from build123d import *

# Parameters (mm, degrees)
SKETCH1_W                      = 40
SKETCH1_H                      = 100
SKETCH1_W_2                    = 34
SKETCH1_H_2                    = 94
BOSS_EXTRUDE1_DEPTH            = 232.9
CUT_EXTRUDE2_REACH             = 283.987
SKETCH8_W                      = 34
SKETCH8_H                      = 16
CUT_EXTRUDE2_DIRECTION_2_DEPTH = 282.986542232
M4_CLEARANCE_HOLE1_D           = 4.5
M4_CLEARANCE_HOLE1_ON_FACE_2_D = 4.5
M4_CLEARANCE_HOLE1_ON_FACE_3_D = 4.5
M4_CLEARANCE_HOLE1_ON_FACE_4_D = 4.5
FILLET1_R                      = 2
F_3_0_3_DIAMETER_HOLE1_D       = 3
F_3_0_3_DIAMETER_HOLE1_DEPTH   = 3


with BuildPart() as part:
    # Sketch1 → Boss-Extrude1 (new body)
    with BuildSketch(Plane.XY.offset(30)):
        Rectangle(SKETCH1_W, SKETCH1_H)
        Rectangle(SKETCH1_W_2, SKETCH1_H_2, mode=Mode.SUBTRACT)
    extrude(amount=BOSS_EXTRUDE1_DEPTH)

    # Sketch8 → Cut-Extrude2 (cut, up to next)
    with BuildSketch(Plane(origin=(0, 50, 0), x_dir=(1, 0, 0), z_dir=(0, 1, 0)), mode=Mode.PRIVATE) as cut_extrude2_sk1:
        with Locations((0, -254.9)):
            Rectangle(SKETCH8_W, SKETCH8_H)
    cut_extrude2_tool1 = extrude(cut_extrude2_sk1.sketch, amount=-CUT_EXTRUDE2_REACH, mode=Mode.PRIVATE) & part.part
    add(cut_extrude2_tool1.solids().sort_by_distance((0, 50, 254.9))[0], mode=Mode.SUBTRACT)

    # Sketch8 → Cut-Extrude2 direction 2 (cut)
    with BuildSketch(Plane(origin=(0, 50, 0), x_dir=(1, 0, 0), z_dir=(0, 1, 0))):
        with Locations((0, -254.9)):
            Rectangle(SKETCH8_W, SKETCH8_H)
    extrude(amount=CUT_EXTRUDE2_DIRECTION_2_DEPTH, mode=Mode.SUBTRACT)

    # M4 Clearance Hole1 (through all)
    with Locations(Plane(origin=(20, 37, 37.5), x_dir=(0, 0, 1), z_dir=(1, 0, 0))):
        with Locations((0, 0), (0, 37), (217.9, 68), (217.9, 31.7), (217.9, -4.6), (0, 74)):
            Hole(M4_CLEARANCE_HOLE1_D / 2)

    # M4 Clearance Hole1 on face 2 (through all)
    with Locations(Plane(origin=(0, 50, 37.5), x_dir=(0, 0, 1), z_dir=(0, 1, 0))):
        with Locations((0, 0)):
            Hole(M4_CLEARANCE_HOLE1_ON_FACE_2_D / 2)

    # M4 Clearance Hole1 on face 3 (through all)
    with Locations(Plane(origin=(-20, -37, 37.5), x_dir=(0, 0, -1), z_dir=(-1, 0, 0))):
        with Locations((0, 0), (0, -37), (0, -74), (-217.9, -6), (-217.9, -42.3), (-217.9, -78.6)):
            Hole(M4_CLEARANCE_HOLE1_ON_FACE_3_D / 2)

    # M4 Clearance Hole1 on face 4 (through all)
    with Locations(Plane(origin=(0, -50, 37.5), x_dir=(0, 0, -1), z_dir=(0, -1, 0))):
        with Locations((0, 0), (-217.9, 0)):
            Hole(M4_CLEARANCE_HOLE1_ON_FACE_4_D / 2)

    # Fillet1
    fillet1_edges = [part.edges().sort_by_distance(p)[0] for p in [
        (17, 48.5, 246.9),
        (-17, 48.5, 246.9),
    ]]
    fillet(fillet1_edges, radius=FILLET1_R)

    # Ø3.0 (3) Diameter Hole1
    with Locations(Plane(origin=(20, 0, 0), x_dir=(0, 0, -1), z_dir=(1, 0, 0))):
        with Locations((-56.45, -45), (-236.45, -39), (-236.45, -45), (-191.45, -39), (-146.45, -39), (-101.45, -39), (-56.45, -39), (-191.45, -45), (-146.45, -45), (-101.45, -45)):
            Hole(F_3_0_3_DIAMETER_HOLE1_D / 2, depth=F_3_0_3_DIAMETER_HOLE1_DEPTH)


solid = part.part
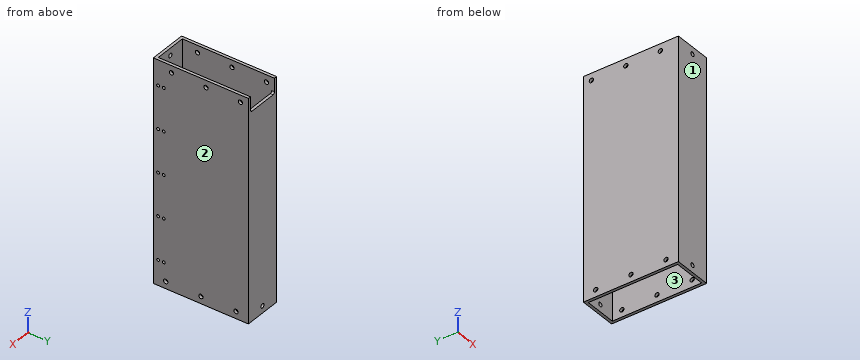
For this review, take the finished solid that the model builds, in its own axes (mm). Face numbers are marked on the shaded views. Give positions to 0.01 mm unless a question says otherwise; leave off trailing zeros. Loops run counter-clockwise (first coordinate to the right, second up) from the corner with the lowest first, then second, coordinate; pieces in that order, holes last. Notation, with made-up numbers: M -14,45.5 L 37,45.5 A17 cw 37,66.5 Z; hole C -16,47 d3. An arc over 180 degrees is marked long. Put each result on its own line as item: value. Start each with the question number.
(1) Wall thickness on L1, parallel to Y at x = 19, z = 255; L2, parallel to X at y = 11, z = 106; L3, parallel to Y at x = -16, z = 216: over which ranges is each line inside the solid? List them lowest first.
(2) Add section C-C, the plane z = 124. Write out the cut boundary in (x, y).
(3) Add section D-D, the plane y = -20. Write out the cut boundary in (x, z).
(4) The part is to be moulded in two halves that separate along Y. For the marked faces 1, 2 and 3, say which applies: +Y half, -Y half, draft (parallel to the pull), parting line (faces both ways), or undercut.
(5) Add section A-A, the plane x = 11.5. Write out the cut boundary in (y, z).
(6) Add section B-B, the plane y = 0. Write out the cut boundary in (x, z), then the cut area to 3 significant figures.
(7) For pin 1 (3.5 mm diameter, centred on y = 5.3, z = 255.4, fed in from +X); pin 2 (2.5 mm diameter, centred on y = -45, z = 236.45, fed in from +X), all flat-tipped, find the tip position at first contact; note any pin that passes through.
Result:
1. L1: y = -50 to -33.21, -28.79 to 3.09, 7.51 to 39.39, 43.81 to 50
1. L2: x = -20 to -17, 17 to 20
1. L3: y = -50 to -47, 47 to 50
2. outline: M -20,-50 L 20,-50 L 20,50 L -20,50 Z; hole M -17,-47 L 17,-47 L 17,47 L -17,47 Z
3. outline: M -20,30 L -17,30 L -17,262.9 L -20,262.9 Z; M 17,30 L 20,30 L 20,262.9 L 17,262.9 Z
4. face 1: -Y half
4. face 2: draft
4. face 3: undercut
5. outline: M -50,30 L -47,30 L -47,262.9 L -50,262.9 Z; M 47,30 L 50,30 L 50,246.9 L 47,246.9 Z
6. outline: M -20,30 L -17,30 L -17,35.25 L -20,35.25 Z; M -20,39.75 L -17,39.75 L -17,262.9 L -20,262.9 Z; M 17,30 L 20,30 L 20,35.25 L 17,35.25 Z; M 17,39.75 L 20,39.75 L 20,262.9 L 17,262.9 Z
6. area: 1,370 mm^2
7. pin 1: passes through
7. pin 2: stops at x = -17
